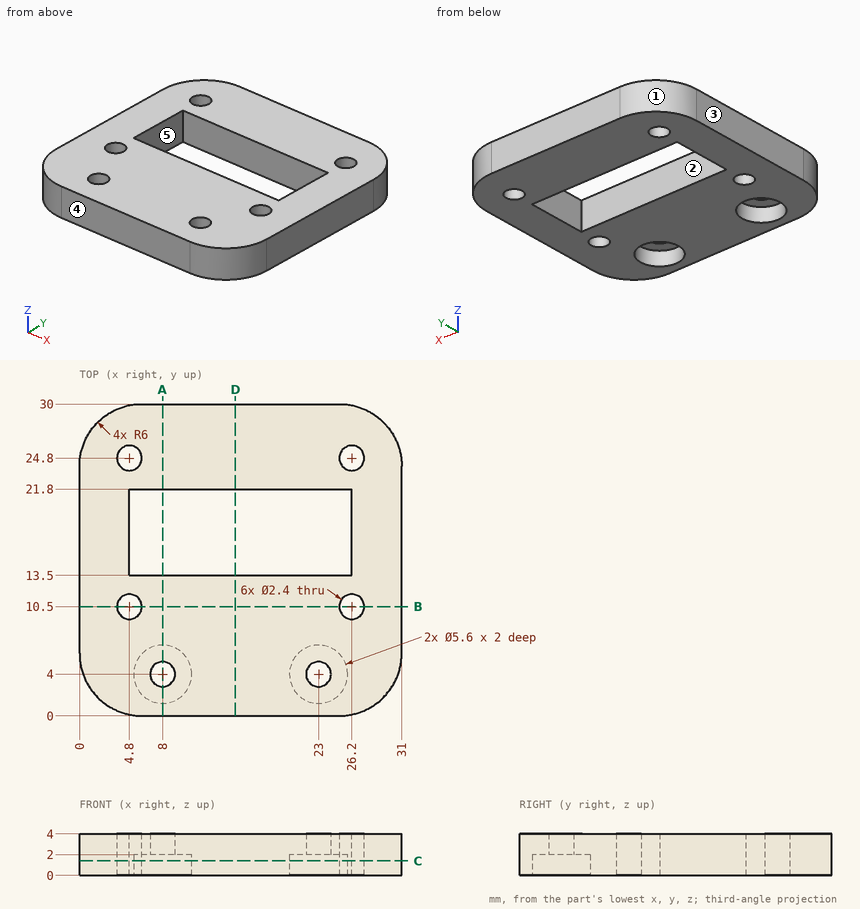
Geometry check sheet. Reference: drawing and pictorial views, mm from the part's lowest x, y, z. A direction names the side the tool comes from. Coordinates: 2 decimals unless noted, no trailing zeros. Write each loop counter-clockwise with the first axis right and the second up, starting at its lowest first coordinate (ties: lowest second). Pieces come first, ordered by that corner, then holes. Notation, with made-up numbers: (88.25, -19.75) - (115.25, -19.75) arc R25 ccw to (115.25, 16.25) - close; hole circle Ø5 at (65, -5.5). An arc over 180 degrees is marked (long way). One line per question, with ' | ' between items. Start each with the question number.
1. Section check B-B (y = 10.5). Enter the section's corners in (x, z), plus the area to 3 significant figures.
2. Access from +Z, -Z, +X, -X, +Y, -Y to the whole of each face (thin tool, end or side, straight path). Record for the marked faces 1 and 2.
3. Material ranges on line 1 along Y through (x, z) = (8, 0.75); line 2 along Y through (x, z) = (20, 1.5); line 3 along X through (y, z) = (17, 2.4), recorded low to high.
4. Gauge pin test, flat ends, axial feed: P1, Ø1.9, axis at x = 8, y = 4, coming from the -Z side; P2, Ø5, axis at x = 8, y = 4, coming from the -Z side. Record the tip position at first contact, or that the pin passes through.
5. Draft check along Y on the marked faces 3, 4 and 5. Enter one of: released by +Y, released by -Y, zero draft, split by the parting line, or undercut.
6. Section check C-C (z = 1.4). Enter the section's corners in (x, y), plus the area to 3 significant figures.
7. Section check A-A (x = 8). Enter the section's corners in (y, z), plus the area to 3 significant figures.
8. Section check D-D (x = 15). Enter the section's corners in (y, z), plus the area to 3 significant figures.
Computed values:
1) outline: (0, 0) - (3.6, 0) - (3.6, 4) - (0, 4) - close; (6, 0) - (25, 0) - (25, 4) - (6, 4) - close; (27.4, 0) - (31, 0) - (31, 4) - (27.4, 4) - close | area: 105 mm²
2) face 1: +Z, -Z, -X, +Y | face 2: +Z, -Z
3) line 1: 0 to 1.2, 6.8 to 13.5, 21.8 to 30 | line 2: 0 to 13.5, 21.8 to 30 | line 3: 0 to 4.8, 26.2 to 31
4) P1: through | P2: z = 2
5) face 3: zero draft | face 4: released by -Y | face 5: undercut
6) outline: (0, 6) arc R6 ccw to (6, 0) - (25, 0) arc R6 ccw to (31, 6) - (31, 24) arc R6 ccw to (25, 30) - (6, 30) arc R6 ccw to (0, 24) - close; hole circle Ø2.4 at (4.8, 10.5); hole circle Ø2.4 at (4.8, 24.8); hole (4.8, 13.5) - (26.2, 13.5) - (26.2, 21.8) - (4.8, 21.8) - close; hole circle Ø5.6 at (8, 4); hole circle Ø5.6 at (23, 4); hole circle Ø2.4 at (26.2, 10.5); hole circle Ø2.4 at (26.2, 24.8) | area: 654 mm²
7) outline: (0, 0) - (1.2, 0) - (1.2, 2) - (2.8, 2) - (2.8, 4) - (0, 4) - close; (5.2, 2) - (6.8, 2) - (6.8, 0) - (13.5, 0) - (13.5, 4) - (5.2, 4) - close; (21.8, 0) - (30, 0) - (30, 4) - (21.8, 4) - close | area: 70.8 mm²
8) outline: (0, 0) - (13.5, 0) - (13.5, 4) - (0, 4) - close; (21.8, 0) - (30, 0) - (30, 4) - (21.8, 4) - close | area: 86.8 mm²
